Design review of the part built by this model. Coordinates are the model's own, in mm. A direction names the side the tool comes from. Give positions to 0.01 mm unless a question says otherwise; leave off trailing zeros. Loops run counter-clockwise (first coordinate to the right, second up) from the corner with the lowest first, then second, coordinate; pieces in that order, holes last. Notation, with made-up numbers: (36.5, 12) -> (52.5, 12) arc R36 cw to (52.5, 50) -> close; hole circle Ø8 at (84, 77). An arc over 180 degrees is marked (long way). Use CSV: the item, a comma, the result in double quotes. Start each with the question number.
Item 1: We need section D-D (z = -44). State the section outline as (x, y) points.
Item 2: We need section A-A (y = -1.3). State the section outline as (x, z) points, plus the area to 3 significant figures.
Item 3: The part is to be moulded in two halves that separate along X. For faces 1 (the face through (165.828, -1.232, -49.846)), 2 (the face through (153.914, -1.232, -48.889)), 3 (the face through (11.704, -1.232, -59.594)), 4 (the face through (81, 0, -28)), say which applies: +X half, -X half, draft (parallel to the pull), parting line (faces both ways), or undercut.
Item 4: Wall thickness on line 1 along X through (y, z) = (-1.65, -33); line 2 along X through (y, z) = (-0.9, -51); line 3 along Z through (x, y) = (121, -1.3): over which ranges is each line inside the solid? List them lowest first. Write a range as from..to.
Item 5: For faces 5 (the face through (25.99, -1.23, -51.29)), 6 (the face through (87.059, -1.232, -49.294)), list the 3-axis set-ups (+Z, -Z, +X, -X, +Y, -Y) from which the entire face can be reached by the end or side of a thin tool; tool diameter is ignored.
Item 6: We need section C-C (x = 75.5). State the section outline as (y, z) points, plus the area to 3 significant figures.
Item 7: We need section B-B (z = -30). State the section outline as (x, y) points, plus the area to 3 significant figures.
from build123d import *

# Parameters (mm, degrees)
F0_R     = 10
F1_DEPTH = 2.5


# Not quite as in the source:
# - a feature names something its author has since deleted; it is built from what else it names


with BuildPart() as f1:
    # F0 (on Front) → F1 (new body)
    with BuildSketch(Plane.XZ):
        with BuildLine():
            ThreePointArc((3.5229699651, 0.2896982716), (2.9467535756, 0.1596707418), (2.3780377062, 0))
            Line((2.3780377062, 0), (4.205058077, 0))
            ThreePointArc((4.205058077, 0), (3.8635532968, 0.1437643709), (3.5229699651, 0.2896982716))
        make_face()
        with BuildLine():
            Line((4.205058077, 0), (2.3780377062, 0))
            ThreePointArc((2.3780377062, 0), (-0.903638288, -1.6292874632), (-3.4998361796, -4.2145788348))
            ThreePointArc((-3.4998361796, -4.2145788348), (-3.5325783371, -4.260242238), (-3.5652547335, -4.3059527224))
            ThreePointArc((-3.5652547335, -4.3059527224), (-10.7285361122, -29.7799444124), (0, -53.9695158351))
            ThreePointArc((0, -53.9695158351), (11.8831829855, -59.6411390335), (25.0231431088, -60.4889571322))
            ThreePointArc((25.0231431088, -60.4889571322), (26.0566140951, -51.1714178585), (33.5999478712, -45.6052058665))
            ThreePointArc((33.5999478712, -45.6052058665), (87.8201274571, -49.2962363), (142.0548581476, -45.8255638994))
            ThreePointArc((142.0548581476, -45.8255638994), (142.7021149729, -45.7037001136), (143.3588035872, -45.6531803752))
            ThreePointArc((143.3588035872, -45.6531803752), (143.5374590966, -45.629232164), (143.7161041215, -45.6052058665))
            ThreePointArc((143.7161041215, -45.6052058665), (143.95071498, -45.6477329831), (144.1850665045, -45.6916667233))
            ThreePointArc((144.1850665045, -45.6916667233), (144.6977602251, -45.7735054296), (145.2015099012, -45.899158479))
            ThreePointArc((145.2015099012, -45.899158479), (154.032538738, -48.9458086752), (161.9085475054, -53.9695158351))
            Line((161.9085475054, -53.9695158351), (169.8591839037, -45.6052058665))
            ThreePointArc((169.8591839037, -45.6052058665), (174.1858351689, -35.1766319754), (173.9545511242, -23.8885155575))
            ThreePointArc((173.9545511242, -23.8885155575), (165.4122565919, -9.5597842761), (151.7413436521, 0))
            ThreePointArc((151.7413436521, 0), (93.1999930381, 2.7960741366), (34.9746532738, -3.8910456933))
            ThreePointArc((34.9746532738, -3.8910456933), (19.3261135001, -4.0311421401), (4.205058077, 0))
        make_face()
        with Locations((15.7105848193, -25)):
            Circle(F0_R, mode=Mode.SUBTRACT)
    extrude(amount=F1_DEPTH)


solid = f1.part
Results found:
1,outline,"(-6.93, -2.5) -> (170.88, -2.5) -> (170.88, 0) -> (-6.93, 0) -> close"
2,outline,"(-3.57, -4.31) arc R39.04 ccw to (0, -53.97) arc R34.78 ccw to (25.02, -60.49) arc R11.7 cw to (33.6, -45.61) arc R412.39 ccw to (142.05, -45.83) arc R6.03 cw to (143.36, -45.65) arc R412.39 ccw to (143.72, -45.61) arc R39.75 cw to (144.19, -45.69) arc R6.03 cw to (145.2, -45.9) arc R39.75 cw to (161.91, -53.97) -> (169.86, -45.61) arc R27.48 ccw to (173.95, -23.89) arc R39.74 ccw to (151.74, 0) arc R362.01 ccw to (34.97, -3.89) arc R58.25 cw to (3.52, 0.29) arc R11.41 ccw to (-3.5, -4.21) arc R39.04 ccw to start; hole circle Ø20 at (15.71, -25)"
2,area,"8,580 mm²"
3,face 1,"+X half"
3,face 2,"undercut"
3,face 3,"parting line"
3,face 4,"draft"
4,line 1,"-10.36..9.71, 21.71..174.51"
4,line 2,"-2.57..26.16, 157.76..164.73"
4,line 3,"-48.03..2.65"
5,face 5,"+Y, -Y"
5,face 6,"-Z, +Y, -Y"
6,outline,"(-2.5, -49.09) -> (0, -49.09) -> (0, 1.77) -> (-2.5, 1.77) -> close"
6,area,"127 mm²"
7,outline,"(-10.71, -2.5) -> (7.05, -2.5) -> (7.05, 0) -> (-10.71, 0) -> close; (24.37, -2.5) -> (174.66, -2.5) -> (174.66, 0) -> (24.37, 0) -> close"
7,area,"420 mm²"
